```python
from build123d import *

# Parameters (mm, degrees)
Y_KSEKLIK_EKSTR_ZYON1_DEPTH = 70
KES_EKSTR_ZYON1_DEPTH       = 41
KES_EKSTR_ZYON1_DEPTH_BACK  = 43


with BuildPart() as part:
    # Çizim1 → Yükseklik-Ekstrüzyon1 (new body)
    with BuildSketch(Plane.XY):
        with BuildLine():
            Line((-16, 20), (16, 20))
            ThreePointArc((16, 20), (18.828427125, 18.828427125), (20, 16))
            Line((20, 16), (20, -16))
            ThreePointArc((20, -16), (18.828427125, -18.828427125), (16, -20))
            Line((16, -20), (-16, -20))
            ThreePointArc((-16, -20), (-18.828427125, -18.828427125), (-20, -16))
            Line((-20, -16), (-20, 16))
            ThreePointArc((-20, 16), (-18.828427125, 18.828427125), (-16, 20))
        make_face()
        with BuildLine():
            Line((-18, 16), (-18, -16))
            ThreePointArc((-18, -16), (-17.414213562, -17.414213562), (-16, -18))
            Line((-16, -18), (16, -18))
            ThreePointArc((16, -18), (17.414213562, -17.414213562), (18, -16))
            Line((18, -16), (18, 16))
            ThreePointArc((18, 16), (17.414213562, 17.414213562), (16, 18))
            Line((16, 18), (-16, 18))
            ThreePointArc((-16, 18), (-17.414213562, 17.414213562), (-18, 16))
        make_face(mode=Mode.SUBTRACT)
    extrude(amount=Y_KSEKLIK_EKSTR_ZYON1_DEPTH)

    # Çizim3 → Kes-Ekstrüzyon1 (cut, two sides: drawn at the far end of the back side and taken through both)
    with BuildSketch(Plane(origin=(0, 0, 0), x_dir=(0, 0, -1), z_dir=(1, 0, 0)).offset(-KES_EKSTR_ZYON1_DEPTH_BACK)):
        Polygon((-70, 20), (-30, -20), (-70, -20), align=None)
    extrude(amount=KES_EKSTR_ZYON1_DEPTH + KES_EKSTR_ZYON1_DEPTH_BACK, mode=Mode.SUBTRACT)


solid = part.part
```
CAD build for the part. Positions are in the model's coordinates, mm. A direction names the side the tool comes from. Give positions to 0.01 mm unless a question says otherwise; leave off trailing zeros. Order: outer loops, then holes, each group sorted by start corner. A loop starts at its lowest first (then second) coordinate and runs counter-clockwise, first axis right, second up.
(1) Flat gauge pin, fed straight in: pin 1 (10 mm diameter, centred on x = -11, y = 12.5, fed in from -Z). Where does the tip first touch, or does it go through?
(2) Drill centre lines: L1, parallel to Y at x = -15.5, z = 14; L2, parallel to Y at x = 5, z = 59.5. Where is each one in solid material? Low to high.
(3) Saw through at A-A, the plane y = -7.5. Give the cut face in (x, z), then the cut area to 3 significant figures.
(4) Saw through at C-C, the plane z = 59. Give the cut face in (x, y).
(5) Tool access for faces 1 (the cylindrical face through (-17.43, -17.4, 16.76)), 2 (the cylindrical face through (-18.859, 18.797, 34.51)): list every direction of +Z, -Z, +X, -X, +Y, -Y with a clear straight run to the whole face (end or side of a thin tool).
(6) Saw through at B-B, the plane x = -7.5. Give the cut face in (y, z), then the cut area to 3 significant figures.
(7) Mould opens along X. For faces 3 (the flat face through (-20, 0, 25)), 4 (the flat face through (0, 20, 35)), 5 (the cylindrical face through (-17.4, 17.43, 33.52)) say: released by +X, released by -X, zero draft, split by the parting line, or undercut.
(8) Saw through at D-D, the plane z = 52. Give the cut face in (x, y), then the cut area to 3 significant figures.
Results found:
1. pin 1: passes through
2. L1: y = -20 to -18, 18 to 20
2. L2: y = 18 to 20
3. outline: (-20, 0) - (-18, 0) - (-18, 42.5) - (-20, 42.5) - close; (18, 0) - (20, 0) - (20, 42.5) - (18, 42.5) - close
3. area: 170 mm2
4. outline: (-20, 9) - (-18, 9) - (-18, 16) arc R2 cw to (-16, 18) - (16, 18) arc R2 cw to (18, 16) - (18, 9) - (20, 9) - (20, 16) arc R4 ccw to (16, 20) - (-16, 20) arc R4 ccw to (-20, 16) - close
5. face 1: +Z, -Z
5. face 2: +Z, -Z, -X, +Y
6. outline: (-20, 0) - (-18, 0) - (-18, 32) - (-20, 30) - close; (18, 0) - (20, 0) - (20, 70) - (18, 68) - close
6. area: 200 mm2
7. face 3: released by -X
7. face 4: zero draft
7. face 5: undercut
8. outline: (-20, 2) - (-18, 2) - (-18, 16) arc R2 cw to (-16, 18) - (16, 18) arc R2 cw to (18, 16) - (18, 2) - (20, 2) - (20, 16) arc R4 ccw to (16, 20) - (-16, 20) arc R4 ccw to (-20, 16) - close
8. area: 139 mm2
